```python
from build123d import *

# Parameters (mm, degrees)
SKETCH_2_W               = 3.5
SKETCH_2_H               = 6
CHAMFER_1_SIZE           = 0.5
SKETCH_4_R               = 10
CUT_EXTRUDE_2_DEPTH      = 1.5
CUT_EXTRUDE_2_DEPTH_BACK = 1.5


with BuildPart() as part:
    # Sketch 2 → Revolve 1 (revolve)
    with BuildSketch(Plane.XY):
        with Locations((19.25, 3)):
            Rectangle(SKETCH_2_W, SKETCH_2_H)
    revolve(axis=Axis((0, 0, 0), (0, 1, 0)))

    # Chamfer 1
    chamfer_1_edges = [part.edges().sort_by_distance(p)[0] for p in [
        (-17.5, 0, 0),
        (-21, 0, 0),
        (-21, 6, 0),
        (-17.5, 6, 0),
    ]]
    chamfer(chamfer_1_edges, length=CHAMFER_1_SIZE)

    # Sketch 4 → Cut-Extrude 2 (cut, two sides)
    with BuildSketch(Plane(origin=(0, 0, 0), x_dir=(0, 0, -1), z_dir=(1, 0, 0))) as cut_extrude_2_sk:
        with Locations((-11.5, 11)):
            Circle(SKETCH_4_R)
        with Locations((11.5, 11)):
            Circle(SKETCH_4_R)
    extrude(amount=CUT_EXTRUDE_2_DEPTH, mode=Mode.SUBTRACT)
    extrude(cut_extrude_2_sk.sketch, amount=-CUT_EXTRUDE_2_DEPTH_BACK, mode=Mode.SUBTRACT)


solid = part.part
```
The listing builds one solid part. Answer for the finished solid, in the listing's coordinates (mm). A direction names the side the tool comes from. Coordinates: 2 decimals unless noted, no trailing zeros. Write each loop counter-clockwise with the first axis right and the second up, starting at its lowest first coordinate (ties: lowest second). Pieces come first, ordered by that corner, then holes. Notation, with made-up numbers: (82, 54.25) - (140, 54.25) arc R14 ccw to (140, 71.25) - close; hole circle Ø11 at (82, 77). An arc over 180 degrees is marked (long way). Return JSON: item names as keys, results as strings. Group by question number.
1. A cutting plane is placed at D-D, the plane y = 4. Determine the outline of the cut face in (x, z), plus the area to 3 significant figures.
2. A cutting plane is placed at C-C, the plane y = 1. Determine the outline of the cut face in (x, z).
3. Determine the mould class of faces 3 (the flat face through (1.5, 5, -18)), 4 (the cylindrical face through (20.03, 3.04, -6.31)), 5 (the flat face through (-1.4, 0, 18.1)) for opening direction Z: released by +Z, released by -Z, zero draft, split by the parting line, or undercut.
4. Given pin 1 (1 mm diameter, centred on x = 11.5, y = 4.5, fed in from +Z); pin 2 (0.8 mm diameter, centred on y = 4, z = -18.5, fed in from +X); pin 3 (2 mm diameter, centred on x = -2.5, y = 4.5, fed in from +Z); pin 4 (12 mm diameter, centred on x = -10.5, z = -9, fed in from +Y), each flat-ended and moving along its own axis, determine where each tip first touches the part or whether it passes through.
5. A cutting plane is placed at A-A, the plane x = 0. Determine the outline of the cut face in (y, z).
6. Straight lines are drawn through the part: L1, parallel to Z at x = 0, y = 2.25; L2, parallel to X at y = 3.5, z = -17.5. For each, find the intervals that lie inside material, in ascending order.
7. Which of the six approach directions +Z, -Z, +X, -X, +Y, -Y give full straight-line access (tool end or side, diameter ignored) to faces 1 (the flat face through (-12, 6, -14)), 2 (the conical face through (17.639, 5.642, 0.367))?
8. A cutting plane is placed at B-B, the plane z = 0. Determine the outline of the cut face in (x, y).
Ans:
{
 "1": {"outline": "circle Ø42 at (0, 0); hole (-1.5, -18.64) - (1.5, -18.64) - (1.5, -17.44) arc R17.5 ccw to (1.5, 17.44) - (1.5, 18.64) - (-1.5, 18.64) - (-1.5, 17.44) arc R17.5 ccw to (-1.5, -17.44) - close", "area": "416 mm²"},
 "2": {"outline": "circle Ø42 at (0, 0); hole circle Ø35 at (0, 0)"},
 "3": {"face 3": "undercut", "face 4": "split by the parting line", "face 5": "zero draft"},
 "4": {"pin 1": "z = 17.89", "pin 2": "x = 10.65", "pin 3": "z = 20.95", "pin 4": "y = 6"},
 "5": {"outline": "(0, -20.5) - (0.5, -21) - (5.5, -21) - (6, -20.5) - (6, -20.16) arc R10 cw to (3, -17.5) - (0.5, -17.5) - (0, -18) - close; (0, 18) - (0.5, 17.5) - (3, 17.5) arc R10 cw to (6, 20.16) - (6, 20.5) - (5.5, 21) - (0.5, 21) - (0, 20.5) - close"},
 "6": {"L1": "-21 to -17.5, 17.5 to 21", "L2": "-11.61 to -1.5, 1.5 to 11.61"},
 "7": {"face 1": "+Z, -Z, +X, -X, +Y", "face 2": "+Y"},
 "8": {"outline": "(-21, 0.5) - (-20.5, 0) - (-18, 0) - (-17.5, 0.5) - (-17.5, 5.5) - (-18, 6) - (-20.5, 6) - (-21, 5.5) - close; (17.5, 0.5) - (18, 0) - (20.5, 0) - (21, 0.5) - (21, 5.5) - (20.5, 6) - (18, 6) - (17.5, 5.5) - close"}
}
